Geometry: final body of the model. Coordinates: model frame, mm. A direction names the side the tool comes from. Give positions to 0.01 mm unless a question says otherwise; leave off trailing zeros. Order: outer loops, then holes, each group sorted by start corner. A loop starts at its lowest first (then second) coordinate and runs counter-clockwise, first axis right, second up. Notation, with made-up numbers: (24, 74.5) -> (49, 74.5) arc R11 cw to (49, 83.5) -> close; hole circle Ø7 at (14.25, 16). An arc over 180 degrees is marked (long way). Write item = value, one per line.
```python
from build123d import *

# Parameters (mm, degrees)
ESQUISSE3_W                  = 6.4
ESQUISSE3_H                  = 6
ENL_V_START                  = 2.5
ESQUISSE5_R                  = 1.6
ENL_V_MAT_EXTRU_1_DEPTH      = 7.5
ENL_V_START_2                = -7
ESQUISSE5_2_R                = 1.6
ENL_V_MAT_EXTRU_2_DEPTH      = 17
R_P_TITION_CIRCULAIRE1_COUNT = 3
ENL_V_MAT_EXTRU_3_DEPTH      = 16


with BuildPart() as part:
    # Esquisse3 → R_volution1 (revolve)
    with BuildSketch(Plane.XY):
        Polygon((9, 9), (0, 9), (0, 0), (17, 0), (17, 2.5), align=None)
        with Locations((3.2, -3)):
            Rectangle(ESQUISSE3_W, ESQUISSE3_H)
    revolve(axis=Axis((0, 0, 0), (0, 1, 0)))

    # Esquisse5 → Enl_v. mat.-Extru.1 (cut, through all)
    with BuildSketch(Plane(origin=(0, 0, 0), x_dir=(1, 0, 0), z_dir=(0, 1, 0)).offset(ENL_V_START)):
        Polygon((1.616580754, 8.747005384), (3.233161507, 11.547005384), (1.616580754, 14.347005384), (-1.616580754, 14.347005384), (-3.233161507, 11.547005384), (-1.616580754, 8.747005384), align=None)
        with Locations((0, 11.547005384)):
            Circle(ESQUISSE5_R, mode=Mode.SUBTRACT)
    enl_v_mat_extru_1 = extrude(amount=ENL_V_MAT_EXTRU_1_DEPTH, mode=Mode.SUBTRACT)

    # Esquisse5_2 → Enl_v. mat.-Extru.2 (cut)
    with BuildSketch(Plane(origin=(0, 0, 0), x_dir=(1, 0, 0), z_dir=(0, 1, 0)).offset(ENL_V_START_2)):
        with Locations((0, 11.547005384)):
            Circle(ESQUISSE5_2_R)
    enl_v_mat_extru_2 = extrude(amount=ENL_V_MAT_EXTRU_2_DEPTH, mode=Mode.SUBTRACT)

    # R_p_tition circulaire1: Enl_v. mat.-Extru.1, Enl_v. mat.-Extru.2 ×3 about axis
    r_p_tition_circulaire1_axis = Axis((0, 0, 0), (0, 1, 0))
    for i in range(1, R_P_TITION_CIRCULAIRE1_COUNT):
        add(enl_v_mat_extru_1.rotate(r_p_tition_circulaire1_axis, i * 360 / R_P_TITION_CIRCULAIRE1_COUNT), mode=Mode.SUBTRACT)
        add(enl_v_mat_extru_2.rotate(r_p_tition_circulaire1_axis, i * 360 / R_P_TITION_CIRCULAIRE1_COUNT), mode=Mode.SUBTRACT)

    # Esquisse6 → Enl_v. mat.-Extru.3 (cut, through all)
    with BuildSketch(Plane(origin=(0, 9, 0), x_dir=(1, 0, 0), z_dir=(0, 1, 0))):
        with BuildLine():
            Line((1.209338662, 2.8), (-1.209338662, 2.8))
            ThreePointArc((-1.209338662, 2.8), (-1.675412946, -2.548625406), (3.05, 0))
            ThreePointArc((3.05, 0), (2.548625406, 1.675412946), (1.209338662, 2.8))
        make_face()
    extrude(amount=-ENL_V_MAT_EXTRU_3_DEPTH, mode=Mode.SUBTRACT)


solid = part.part
```
1) Line query: line 1 (Z direction, x = 0, y = 2); line 2 (Z direction, x = 0, y = -4); line 3 (X direction, y = -3.5, z = 0.5). Output: solid intervals per line, ascending. Write a range as from..to.
Check sheet entries:
line_1 = -17..-13.15, -9.95..-2.8, 3.05..17
line_2 = -6.4..-2.8, 3.05..6.4
line_3 = -6.38..-3.01, 3.01..6.38
2) Reachability of faces 3 (the face through (-12.41, 4.05, 4.35)), 4 (the face through (-5.08, -2.96, 3.89)), 5 (the face through (0, 2, -2.8)) from +Z, -Z, +X, -X, +Y, -Y: full face, straight path, thin tool, end or side. Return the list, or none.
Check sheet entries:
face_3 = +Y
face_4 = -Y
face_5 = +Y, -Y
3) First-contact query: P1, Ø4, axis at x = -10, z = 5.77, coming from the +Y side; P2, Ø6, axis at x = -8, z = 5.5, coming from the -Y side; P3, Ø1.7, axis at x = -0.5, y = 4, coming from the +Z side. Flat tips, straight axial feed; report the tip coordinate or a pass-through.
Check sheet entries:
P1 = 2.5
P2 = 0
P3 = 16.19
4) Section query B-B (y = 7). Output: boundary loops of the cut face in (x, z).
Check sheet entries:
outline = (-11.07, 2.97) arc R11.46 ccw to (-2.96, -11.07) -> (-1.62, -8.75) -> (1.62, -8.75) -> (2.96, -11.07) arc R11.46 ccw to (11.07, 2.97) -> (8.38, 2.97) -> (6.77, 5.77) -> (8.11, 8.1) arc R11.46 ccw to (-8.11, 8.1) -> (-6.77, 5.77) -> (-8.38, 2.97) -> close; hole (-1.21, -2.8) -> (1.21, -2.8) arc R3.05 ccw (long way) to start
5) Section query A-A (x = 0). Output: boundary loops of the cut face in (y, z), plus the area to 3 significant figures.
Check sheet entries:
outline = (-6, -6.4) -> (0, -6.4) -> (0, -9.95) -> (2.5, -9.95) -> (2.5, -8.75) -> (9, -8.75) -> (9, -2.8) -> (-6, -2.8) -> close; (-6, 3.05) -> (9, 3.05) -> (9, 9) -> (2.5, 17) -> (0, 17) -> (0, 6.4) -> (-6, 6.4) -> close; (0, -17) -> (2.5, -17) -> (4.66, -14.35) -> (2.5, -14.35) -> (2.5, -13.15) -> (0, -13.15) -> close
area = 210 mm²
6) Mould query, pull axis Z, two halves, no side actions, for faces 1 (the face through (9.139, 1.268, -14.334)), 2 (the face through (-10, 4, 8.574)). Classes: +Z half, -Z half, draft (parallel to the pull), parting line (faces both ways), or undercut.
Check sheet entries:
face_1 = parting line
face_2 = undercut
7) Section query D-D (y = -1.5). Output: boundary loops of the cut face in (x, z), plus the area to 3 significant figures.
Check sheet entries:
outline = circle Ø12.8 at (0, 0); hole (-1.21, -2.8) -> (1.21, -2.8) arc R3.05 ccw (long way) to start
area = 99.9 mm²
8) Section query C-C (y = 4). Output: boundary loops of the cut face in (x, z).
Check sheet entries:
outline = circle Ø30.31 at (0, 0); hole (-13.23, 5.77) -> (-11.62, 2.97) -> (-8.38, 2.97) -> (-6.77, 5.77) -> (-8.38, 8.57) -> (-11.62, 8.57) -> close; hole (-3.23, -11.55) -> (-1.62, -14.35) -> (1.62, -14.35) -> (3.23, -11.55) -> (1.62, -8.75) -> (-1.62, -8.75) -> close; hole (-1.21, -2.8) -> (1.21, -2.8) arc R3.05 ccw (long way) to start; hole (6.77, 5.77) -> (8.38, 2.97) -> (11.62, 2.97) -> (13.23, 5.77) -> (11.62, 8.57) -> (8.38, 8.57) -> close
